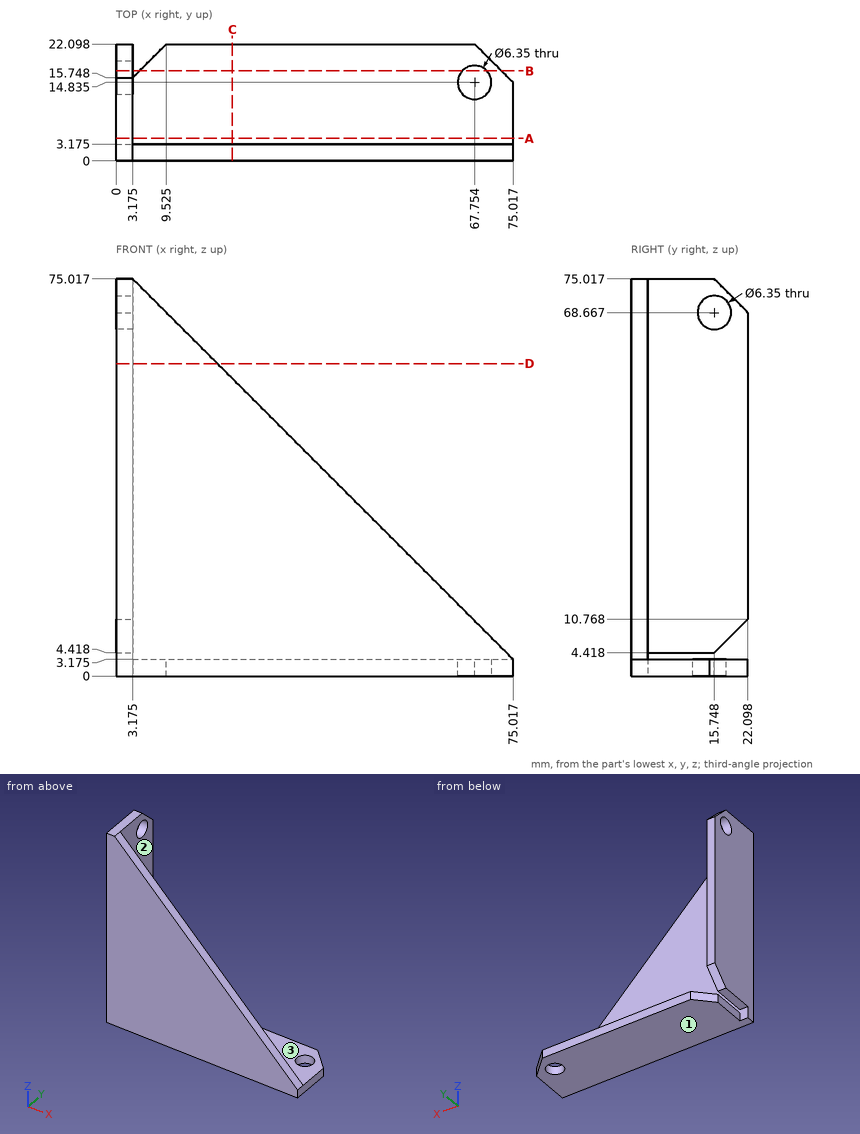
Check sheet for the drawn part. Datum: minimum x, y, z corner. Units: mm. A direction names the side the tool comes from. Coordinates: 2 decimals unless noted, no trailing zeros. Loops run counter-clockwise (first coordinate to the right, second up) from the corner with the lowest first, then second, coordinate; pieces in that order, holes last. Notation, with made-up numbers: (-8.75, 41) -> (28.25, 41) arc R25 cw to (28.25, 74) -> close; hole circle Ø6 at (-7.5, 87). An arc over 180 degrees is marked (long way). Answer as a JSON object with one key per item and string values. Group by question number.
Item 1: Sectioned sample at B-B on y = 17. Record the boundary of the cut face in (x, z) (1 decimal), plus the area to 3 significant figures.
Item 2: Tool access check on the marked faces 1, 2 and 3. Record the directions out of +Z, -Z, +X, -X, +Y, -Y that give a thin tool (end or side, any length) a straight path to the whole face; none if there is none.
Item 3: Sectioned sample at C-C on x = 22. Record the boundary of the cut face in (y, z) (3 decimals).
Item 4: Sectioned sample at A-A on y = 4.25. Record the boundary of the cut face in (x, z) (3 decimals).
Item 5: Scan line: probe 1 along X at (y, z) = (7.25, 10) (3 decimals). Record every from-to range of solid material in increasing order.
Item 6: Depth check by flat-ended pin: pin 1 (3 mm diameter, centred on x = 48, z = 34, fed in from -Y); pin 2 (12 mm diameter, centred on x = 34, y = 3, fed in from -Z); pin 3 (8 mm diameter, centred on y = 4, z = 37.5, fed in from +X); pin 4 (4 mm diameter, centred on x = 23, y = 6.5, fed in from +Z) (3 decimals). Enter the tip coordinate at first touch or a pass-through.
Item 7: Sectioned sample at D-D on z = 59. Record the boundary of the cut face in (x, y) (3 decimals), plus the area to 3 significant figures.
Evaluation:
{
 "1": {"outline": "(0, 5.7) -> (3.2, 5.7) -> (3.2, 65.7) -> (0, 65.7) -> close; (0, 71.6) -> (3.2, 71.6) -> (3.2, 73.8) -> (0, 73.8) -> close; (4.4, 0) -> (65.4, 0) -> (65.4, 3.2) -> (4.4, 3.2) -> close; (70.1, 0) -> (72.9, 0) -> (72.9, 3.2) -> (70.1, 3.2) -> close", "area": "400 mm²"},
 "2": {"face 1": "-Z, +X, -X, +Y, -Y", "face 2": "+Z, +X, +Y", "face 3": "+Z, +X, -X, +Y"},
 "3": {"outline": "(0, 0) -> (22.098, 0) -> (22.098, 3.175) -> (3.175, 3.175) -> (3.175, 56.192) -> (0, 56.192) -> close"},
 "4": {"outline": "(0, 4.418) -> (3.175, 4.418) -> (3.175, 75.017) -> (0, 75.017) -> close; (3.175, 0) -> (75.017, 0) -> (75.017, 3.175) -> (3.175, 3.175) -> close"},
 "5": {"probe 1": "x = 0 to 3.175"},
 "6": {"pin 1": "passes through", "pin 2": "stops at z = 0", "pin 3": "stops at x = 44.61", "pin 4": "stops at z = 3.175"},
 "7": {"outline": "(0, 0) -> (19.192, 0) -> (19.192, 3.175) -> (3.175, 3.175) -> (3.175, 22.098) -> (0, 22.098) -> close", "area": "121 mm²"}
}
